The model under review builds one solid part; all positions refer to its coordinate system, in mm. Round coordinates to 2 decimals unless told otherwise and drop trailing zeros. Loops run counter-clockwise (first coordinate to the right, second up) from the corner with the lowest first, then second, coordinate; pieces in that order, holes last. Notation, with made-up numbers: (33, -24) -> (67, -24) arc R16 ccw to (67, -3) -> close; hole circle Ø10 at (43.25, -23.5). An arc over 180 degrees is marked (long way). Write each question's results on one line, items separated by ' | '. Start each with the question number.
Item 1: For L1, parallel to Z at x = 0, y = 3.85; L2, parallel to Y at x = -3.25, z = -10, list the stretches that pass through material, from the lowest coordinate up. Write a range as from..to.
Item 2: We need section C-C (y = 4.85). Give the boundary of the cut face in (x, z).
Item 3: We need section B-B (z = 0). Give the boundary of the cut face in (x, y), and give its area (3 significant figures).
Item 4: We need section A-A (x = 0). Give the boundary of the cut face in (y, z), and give its area (3 significant figures).
Item 5: Clearance check with a flat-ended pin moving along its axis: pin 1 Ø1 at (y, z) = (4.5, 1) entering from +X. State where the tip first meets the part, or that it passes through.
Item 6: Mouldability with a two-part tool opening along Z and no side actions: class faces 1 (the flat face through (0, 0.5, 10)), 2 (the cylindrical face through (-0.867, 3.039, 3.905)), 3 (the cylindrical face through (4.38, 3.11, -8.43)) as pulls with the +Z half, pulls with the -Z half, needs draft (parallel to the pull), parting line crosses it, or undercut.
Autodesk Inventor part; units mm, degrees
ref_plane "YZ Plane" through (0, 0, 0) normal (1, 0, 0) x (0, 1, 0)
ref_plane "XZ Plane" through (0, 0, 0) normal (0, 1, 0) x (-1, 0, 0)
ref_plane "XY Plane" through (0, 0, 0) normal (0, 0, 1) x (1, 0, 0)
sketch "スケッチ1" plane through (0, 0, 0) normal (0, 0, 1) x (1, 0, 0)
  line L0 (4, 0) -> (4, 6)
  line L1 (4, 6) -> (9.5, 6)
  line L2 (9.5, 6) -> (9.5, 0.5)
  line L3 (9.5, 0.5) -> (11, 0.5)
  line L4 (11, 0.5) -> (11, 0)
  line L5 (11, 0) -> (4, 0)
  line L6 (0, 0) -> (0, 6.1022) construction
  dimension "d0" = 4
  dimension "d1" = 6
  dimension "d2" = 0.5
  dimension "d3" = 9.5
  dimension "d4" = 11
revolve "回転1" add sketch "スケッチ1" angle 360 about axis through (0, 0, 0) along (0, 1, 0)
chamfer "面取り1" distance 0.2 angle 45 5 edges at (-4, 6, 0) (-9.5, 6, 0) (-11, 0.5, 0) (-11, 0, 0) (-4, 0, 0)
properties part number "ベアリングフランジ付き"
Here are the results:
1) L1: z = -9.5..-4, 4..9.5 | L2: y = 0..0.5
2) outline: circle Ø19 at (0, 0); hole circle Ø8 at (0, 0)
3) outline: (-11, 0.2) -> (-10.8, 0) -> (-4.2, 0) -> (-4, 0.2) -> (-4, 5.8) -> (-4.2, 6) -> (-9.3, 6) -> (-9.5, 5.8) -> (-9.5, 0.5) -> (-10.8, 0.5) -> (-11, 0.3) -> close; (4, 0.2) -> (4.2, 0) -> (10.8, 0) -> (11, 0.2) -> (11, 0.3) -> (10.8, 0.5) -> (9.5, 0.5) -> (9.5, 5.8) -> (9.3, 6) -> (4.2, 6) -> (4, 5.8) -> close | area: 67.3 mm2
4) outline: (0, -10.8) -> (0.2, -11) -> (0.3, -11) -> (0.5, -10.8) -> (0.5, -9.5) -> (5.8, -9.5) -> (6, -9.3) -> (6, -4.2) -> (5.8, -4) -> (0.2, -4) -> (0, -4.2) -> close; (0, 4.2) -> (0.2, 4) -> (5.8, 4) -> (6, 4.2) -> (6, 9.3) -> (5.8, 9.5) -> (0.5, 9.5) -> (0.5, 10.8) -> (0.3, 11) -> (0.2, 11) -> (0, 10.8) -> close | area: 67.3 mm2
5) pin 1: stops at x = 9.49
6) face 1: needs draft | face 2: undercut | face 3: parting line crosses it
